```python
from build123d import *

# Parameters (mm, degrees)
F1_DEPTH  = 5
F3_DEPTH  = 25
F5_DEPTH  = 25
F6_R      = 2.5
F7_DEPTH  = 25
F8_R      = 2.5
F9_DEPTH  = 25
F10_W     = 16
F10_H     = 30
F11_DEPTH = 2
F13_R     = 2.5
F14_DEPTH = 10


with BuildPart() as f1:
    # F0 (on Front) → F1 (new body, symmetric)
    with BuildSketch(Plane.XZ):
        Polygon((0, 50), (0, 0), (2, 0), (2, 10), (2, 40), (2, 50), align=None)
    extrude(amount=F1_DEPTH, both=True)


with BuildPart() as f1b:
    # F0 (on Front) → F1, piece 2 (new body, symmetric)
    with BuildSketch(Plane.XZ):
        Polygon((18, 40), (18, 10), (18, 0), (20, 0), (20, 50), (18, 50), align=None)
    extrude(amount=F1_DEPTH, both=True)


with BuildPart() as f3_tool:
    # F2 (on face) → F3 (new body)
    with BuildSketch(Plane(origin=(0, 0, 0), x_dir=(0, -1, 0), z_dir=(-1, 0, 0))):
        with BuildLine():
            ThreePointArc((5, 5), (3.5355339059, 1.4644660941), (0, 0))
            Line((0, 0), (5, 0))
            Line((5, 0), (5, 5))
        make_face()
        with BuildLine():
            ThreePointArc((0, 0), (-3.5355339059, 1.4644660941), (-5, 5))
            Line((-5, 5), (-5, 0))
            Line((-5, 0), (0, 0))
        make_face()
    extrude(amount=-F3_DEPTH)


with BuildPart() as f1_1:
    add(f1.part)

    # F3: cut by f3_tool
    add(f3_tool.part, mode=Mode.SUBTRACT)


with BuildPart() as f1b_1:
    add(f1b.part)

    # F3: cut by f3_tool
    add(f3_tool.part, mode=Mode.SUBTRACT)


with BuildPart() as f5_tool:
    # F4 (on face) → F5 (new body)
    with BuildSketch(Plane(origin=(0, 0, 0), x_dir=(0, -1, 0), z_dir=(-1, 0, 0))):
        with BuildLine():
            ThreePointArc((-5, 45), (-3.5355339059, 48.5355339059), (0, 50))
            Line((0, 50), (-5, 50))
            Line((-5, 50), (-5, 45))
        make_face()
        with BuildLine():
            ThreePointArc((0, 50), (3.5355339059, 48.5355339059), (5, 45))
            Line((5, 45), (5, 50))
            Line((5, 50), (0, 50))
        make_face()
    extrude(amount=-F5_DEPTH)


with BuildPart() as f1_2:
    add(f1_1.part)

    # F5: cut by f5_tool
    add(f5_tool.part, mode=Mode.SUBTRACT)


with BuildPart() as f1b_2:
    add(f1b_1.part)

    # F5: cut by f5_tool
    add(f5_tool.part, mode=Mode.SUBTRACT)


with BuildPart() as f7_tool:
    # F6 (on face) → F7 (new body)
    with BuildSketch(Plane(origin=(0, 0, 0), x_dir=(0, -1, 0), z_dir=(-1, 0, 0))):
        with Locations((0, 45)):
            Circle(F6_R)
    extrude(amount=-F7_DEPTH)


with BuildPart() as f1_3:
    add(f1_2.part)

    # F7: cut by f7_tool
    add(f7_tool.part, mode=Mode.SUBTRACT)


with BuildPart() as f1b_3:
    add(f1b_2.part)

    # F7: cut by f7_tool
    add(f7_tool.part, mode=Mode.SUBTRACT)


with BuildPart() as f9_tool:
    # F8 (on face) → F9 (new body)
    with BuildSketch(Plane(origin=(0, 0, 0), x_dir=(0, -1, 0), z_dir=(-1, 0, 0))):
        with Locations((0, 5)):
            Circle(F8_R)
    extrude(amount=-F9_DEPTH)


with BuildPart() as f1_4:
    add(f1_3.part)

    # F9: cut by f9_tool
    add(f9_tool.part, mode=Mode.SUBTRACT)


with BuildPart() as f1b_4:
    add(f1b_3.part)

    # F9: cut by f9_tool
    add(f9_tool.part, mode=Mode.SUBTRACT)


with BuildPart() as f11:
    # F10 (on face) → F11 (new body)
    with BuildSketch(Plane.XZ.offset(5)):
        with Locations((10, 25)):
            Rectangle(F10_W, F10_H)
    extrude(amount=-F11_DEPTH)


with BuildPart() as f1_5:
    add(f1_4.part)

    # F12: union F1b, F11
    add(f1b_4.part)
    add(f11.part)

    # F13 (on face) → F14 (cut)
    with BuildSketch(Plane.YZ.offset(20)):
        with BuildLine():
            ThreePointArc((-5, 45), (-3.5355339059, 48.5355339059), (0, 50))
            Line((0, 50), (-5, 50))
            Line((-5, 50), (-5, 45))
        make_face()
        with BuildLine():
            ThreePointArc((0, 50), (3.5355339059, 48.5355339059), (5, 45))
            Line((5, 45), (5, 50))
            Line((5, 50), (0, 50))
        make_face()
        with Locations((0, 45)):
            Circle(F13_R)
        with BuildLine():
            ThreePointArc((5, 5), (3.5355339059, 1.4644660941), (0, 0))
            Line((0, 0), (5, 0))
            Line((5, 0), (5, 5))
        make_face()
        with BuildLine():
            ThreePointArc((0, 0), (-3.5355339059, 1.4644660941), (-5, 5))
            Line((-5, 5), (-5, 0))
            Line((-5, 0), (0, 0))
        make_face()
        with Locations((0, 5)):
            Circle(F13_R)
    extrude(amount=-F14_DEPTH, mode=Mode.SUBTRACT)


solid = f1_5.part
```
Model file for the job. Use its own axes, mm. A direction names the side the tool comes from. Coordinates: 2 decimals unless noted, no trailing zeros. Loops run counter-clockwise (first coordinate to the right, second up) from the corner with the lowest first, then second, coordinate; pieces in that order, holes last. Notation, with made-up numbers: (26, -17) - (68, -17) arc R17 ccw to (68, -3) - close; hole circle Ø3 at (-37, -2). An arc over 180 degrees is marked (long way). Write item = value, one per line. Start each with the question number.
Item 1: 3-axis set-ups, long thin cutter, end or side, ignore diameter. For faces 4 (the face through (10, -4, 40)), 5 (the face through (0.99, 0.54, 42.56)): which of +Z, -Z, +X, -X, +Y, -Y reach the whole face in a straight line?
Item 2: Drop flat-ended pins along their axis: pin 1 Ø2 at (x, y) = (10, -3.5) entering from -Z; pin 2 Ø1 at (x, y) = (9, -4.5) entering from +Z. Give the stop position or say it passes through.
Item 3: Saw through at B-B, the plane z = 9. List the corners of the cut face in (x, y).
Item 4: Pull direction Z, two halves, no side cores. Call faces 1 (the face through (18.99, 0.54, 42.56)), 2 (the face through (10, -4, 10)), 3 (the face through (10, -3, 25)): +Z half, -Z half, draft (parallel to the pull), parting line (faces both ways), or undercut.
Item 5: Wall check: probe 1 along Z at (x, y) = (19, 0); probe 2 along X at (y, z) = (4, 6); probe 3 along Z at (x, y) = (18.5, 1.5). Give the ranges that are in metal, low to high. Write a range as [from, to].
Item 6: Saw through at A-A, the plane y = 3. List the corners of the cut face in (x, z), then the cut area to 3 significant figures.
Item 7: Saw through at D-D, the plane z = 22.5. List the corners of the cut face in (x, y), then the cut area to 3 significant figures.
Item 8: Saw through at C-C, the plane y = -1. List the corners of the cut face in (x, z), then the cut area to 3 significant figures.
Answers:
q1.face_4 = +Z, +Y, -Y
q1.face_5 = +X, -X
q2.pin_1 = 10
q2.pin_2 = 40
q3.outline = (0, -5) - (2, -5) - (2, 5) - (0, 5) - close; (18, -5) - (20, -5) - (20, 5) - (18, 5) - close
q4.face_1 = undercut
q4.face_2 = -Z half
q4.face_3 = draft
q5.probe_1 = [0, 2.5], [7.5, 42.5], [47.5, 50]
q5.probe_2 = [0, 2], [18, 20]
q5.probe_3 = [0.23, 3], [7, 43], [47, 49.77]
q6.outline = (0, 1) - (2, 1) - (2, 49) - (0, 49) - close; (18, 1) - (20, 1) - (20, 49) - (18, 49) - close
q6.area = 192 mm2
q7.outline = (0, -5) - (20, -5) - (20, 5) - (18, 5) - (18, -3) - (2, -3) - (2, 5) - (0, 5) - close
q7.area = 72.0 mm2
q8.outline = (0, 0.1) - (2, 0.1) - (2, 2.71) - (0, 2.71) - close; (0, 7.29) - (2, 7.29) - (2, 42.71) - (0, 42.71) - close; (0, 47.29) - (2, 47.29) - (2, 49.9) - (0, 49.9) - close; (18, 0.1) - (20, 0.1) - (20, 2.71) - (18, 2.71) - close; (18, 7.29) - (20, 7.29) - (20, 42.71) - (18, 42.71) - close; (18, 47.29) - (20, 47.29) - (20, 49.9) - (18, 49.9) - close
q8.area = 163 mm2
